Source: CAD feature listing. Evaluate the final solid. Frame: model axes, mm. A direction names the side the tool comes from. Coordinates: 2 decimals unless noted, no trailing zeros.
Item 1: Line query: probe 1 along X at (y, z) = (477, 56.5); probe 2 along X at (y, z) = (487, 73). Output: solid intervals per line, ascending.
Item 2: Pull-direction query (Y, two-part tool) for faces 6 (the flat face through (386.799, 482.244, 45.072)), 7 (the flat face through (1174, 139.7, 45)), 8 (the flat face through (1219.2, 393, 45)), 9 (the flat face through (1137.201, 25.756, 45.072)); classes: +Y half, -Y half, draft (parallel to the pull), parting line (faces both ways), or undercut.
Item 3: Section query A-A, the plane z = 38.5. State how many separate pieces and enclosed holes the cut face has, then the cut area to 3 significant figures.
Item 4: Reachability of faces 1 (the flat face through (1212.299, 482.244, 45.072)), 2 (the flat face through (1369, 508, 44)), 3 (the flat face through (0, 250, 44)), 4 (the flat face through (1174, 88.9, 45)), 5 (the flat face through (311.701, 25.756, 45.072)) from +Z, -Z, +X, -X, +Y, -Y: full face, straight path, thin tool, end or side. Return the list, or none.
Item 5: Pin query (flat end, axial travel): pin 1 Ø12 at (x, z) = (363.5, 59) entering from +Y; pin 2 Ø18.5 at (x, z) = (1181.5, 47.5) entering from -Y. Return the tip coordinate at first contact, or that it passes through.
```python
from build123d import *

# Parameters (mm, degrees)
F0_W     = 1524
F0_H     = 508
F1_DEPTH = 88.9
F2_W     = 88.9
F2_H     = 50.8
F3_DEPTH = 88.9


with BuildPart() as f1:
    # F0 (on Top) → F1 (new body)
    with BuildSketch(Plane.XY):
        with Locations((762, 254)):
            Rectangle(F0_W, F0_H)
    extrude(amount=F1_DEPTH)

    # F2 (on face) → F3 (cut, through all)
    with BuildSketch(Plane.XY.offset(88.9)):
        Polygon((318.411819, 50.8), (304.8, 0), (393.7, 0), (380.088181, 50.8), align=None)
        with Locations((349.25, 114.3)):
            Rectangle(F2_W, F2_H)
        Polygon((1143.911819, 50.8), (1130.3, 0), (1219.2, 0), (1205.588181, 50.8), align=None)
        with Locations((1174.75, 114.3)):
            Rectangle(F2_W, F2_H)
        Polygon((318.411819, 457.2), (380.088181, 457.2), (393.7, 508), (304.8, 508), align=None)
        with Locations((1174.75, 393.7)):
            Rectangle(F2_W, F2_H)
        with Locations((349.25, 393.7)):
            Rectangle(F2_W, F2_H)
        Polygon((1205.588181, 457.2), (1219.2, 508), (1130.3, 508), (1143.911819, 457.2), align=None)
    extrude(amount=-F3_DEPTH, mode=Mode.SUBTRACT)


solid = f1.part
```
Verdict:
1. probe 1: x = 0 to 313.11, 385.39 to 1138.61, 1210.89 to 1524
1. probe 2: x = 0 to 310.43, 388.07 to 1135.93, 1213.57 to 1524
2. face 6: +Y half
2. face 7: undercut
2. face 8: undercut
2. face 9: -Y half
3. separate pieces: 1
3. enclosed holes: 4
3. area: 741,000 mm2
4. face 1: +Z, -Z, +Y
4. face 2: +Z, -Z, +X, -X, +Y
4. face 3: +Z, -Z, -X, +Y, -Y
4. face 4: +Z, -Z
4. face 5: +Z, -Z, -Y
5. pin 1: stops at y = 457.2
5. pin 2: stops at y = 50.8
